The listing builds one solid part. Answer for the finished solid, in the listing's coordinates (mm). A direction names the side the tool comes from. Coordinates: 2 decimals unless noted, no trailing zeros. Order: outer loops, then holes, each group sorted by start corner. A loop starts at its lowest first (then second) coordinate and runs counter-clockwise, first axis right, second up. Notation, with made-up numbers: (70, 70.5) -> (83, 70.5) arc R23 ccw to (83, 78.5) -> close; hole circle Ø2 at (86.25, 31). An arc over 180 degrees is marked (long way). Write item = value, one per line.
from build123d import *

# Parameters (mm, degrees)
F1_DEPTH = 750
F2_DEPTH = 10
F6_R     = 5


# Not quite as in the source:
# - a feature of the source that left no trace in its solid (it failed there, or was rolled back) is left out


with BuildPart() as f1:
    # F0 (on Right) → F1 (new body)
    with BuildSketch(Plane.YZ):
        with BuildLine():
            Line((-213.512294728, 30), (-230, 30))
            Line((-230, 30), (-230, -30))
            Line((-230, -30), (-220, -30))
            Line((-220, -30), (-220, 25.1203247649))
            ThreePointArc((-220, 25.1203247649), (-216.7698785064, 27.5784184345), (-213.512294728, 30))
        make_face()
        with BuildLine():
            ThreePointArc((230, 30), (0, 110), (-230, 30))
            Line((-230, 30), (-213.512294728, 30))
            ThreePointArc((-213.512294728, 30), (0, 100), (213.512294728, 30))
            Line((213.512294728, 30), (230, 30))
        make_face()
        with BuildLine():
            Line((230, -30), (230, 30))
            Line((230, 30), (213.512294728, 30))
            ThreePointArc((213.512294728, 30), (216.7698785064, 27.5784184345), (220, 25.1203247649))
            Line((220, 25.1203247649), (220, -30))
            Line((220, -30), (230, -30))
        make_face()
    extrude(amount=F1_DEPTH)

    # F0 (on Right) → F2 (join)
    with BuildSketch(Plane.YZ):
        with BuildLine():
            ThreePointArc((230, 30), (0, 110), (-230, 30))
            Line((-230, 30), (-213.512294728, 30))
            ThreePointArc((-213.512294728, 30), (0, 100), (213.512294728, 30))
            Line((213.512294728, 30), (230, 30))
        make_face()
        with BuildLine():
            Line((-213.512294728, 30), (-230, 30))
            Line((-230, 30), (-230, -30))
            Line((-230, -30), (-220, -30))
            Line((-220, -30), (-220, 25.1203247649))
            ThreePointArc((-220, 25.1203247649), (-216.7698785064, 27.5784184345), (-213.512294728, 30))
        make_face()
        with BuildLine():
            Line((213.512294728, 30), (-213.512294728, 30))
            ThreePointArc((-213.512294728, 30), (-216.7698785064, 27.5784184345), (-220, 25.1203247649))
            Line((-220, 25.1203247649), (-220, -30))
            Line((-220, -30), (220, -30))
            Line((220, -30), (220, 25.1203247649))
            ThreePointArc((220, 25.1203247649), (216.7698785064, 27.5784184345), (213.512294728, 30))
        make_face()
        with BuildLine():
            ThreePointArc((213.512294728, 30), (0, 100), (-213.512294728, 30))
            Line((-213.512294728, 30), (213.512294728, 30))
        make_face()
        with BuildLine():
            Line((230, -30), (230, 30))
            Line((230, 30), (213.512294728, 30))
            ThreePointArc((213.512294728, 30), (216.7698785064, 27.5784184345), (220, 25.1203247649))
            Line((220, 25.1203247649), (220, -30))
            Line((220, -30), (230, -30))
        make_face()
    extrude(amount=F2_DEPTH)

    # F4: F1 across plane


with BuildPart() as f1_1:
    add(f1.part)
    add(f1.part.mirror(Plane.YZ.offset(375)))

    # F6
    f6_edges = [f1_1.edges().sort_by_distance(p)[0] for p in [
        (750, 0, 110),
        (375, 230, 30),
        (0, 0, 110),
        (375, -230, 30),
        (0, -230, 0),
        (750, -230, 0),
        (0, 230, 0),
        (750, 230, 0),
    ]]
    fillet(f6_edges, radius=F6_R)


solid = f1_1.part
Q1. The mould has two halves that part along X. Classify faces 3 (the face through (370, 230, -2)), 4 (the face through (750, -3, 23)), 5 (the face through (10, -3, 21)): released by +X, released by -X, zero draft, split by the parting line, or undercut.
The answers:
face_3 = zero draft
face_4 = released by +X
face_5 = undercut
Q2. Section A-A, the plane z = -9 is taken. Give the vertices of the cut face in (x, y).
The answers:
outline = (0, -225) arc R5 ccw to (5, -230) -> (745, -230) arc R5 ccw to (750, -225) -> (750, 225) arc R5 ccw to (745, 230) -> (5, 230) arc R5 ccw to (0, 225) -> close; hole (10, -220) -> (740, -220) -> (740, 220) -> (10, 220) -> close
Q3. Each of these flat-tipped pins is pushed along its axis until it touches: pin 1 Ø1 at (x, y) = (446.5, 105.5) entering from -Z; pin 2 Ø4 at (x, y) = (369.5, -52.5) entering from -Z; pin 3 Ø2 at (x, z) = (271, 29.5) entering from +Y. Where does it stop, or does it pass through?
The answers:
pin_1 = 84.07
pin_2 = 95.86
pin_3 = 229.91
Q4. A tool of negligible diameter and unlimited length cuts with its end or side. For faces 1 (the face through (373, -223, -30)), 2 (the face through (740, -3, 21)), from which of +Z, -Z, +X, -X, +Y, -Y can it reach the whole face along a straight path? Write none if from no direction.
The answers:
face_1 = -Z, +X, -X, +Y, -Y
face_2 = -Z
Q5. Find the intervals of material crossed by line 1 along X through (y, z) = (127.5, 16.5); line 2 along Y through (x, z) = (384.5, 9); line 3 along Y through (x, z) = (662.5, 37.5), in increasing order.
The answers:
line_1 = 0 to 10, 740 to 750
line_2 = -230 to -220, 220 to 230
line_3 = -220.19 to -202.91, 202.91 to 220.19
